Read the model definition and answer for the solid it produces. Units are mm, in the model's axes. Face numbers are marked on the shaded views. A direction names the side the tool comes from. Coordinates: 2 decimals unless noted, no trailing zeros. Write each loop counter-clockwise with the first axis right and the second up, starting at its lowest first coordinate (ties: lowest second). Pieces come first, ordered by that corner, then holes. Notation, with made-up numbers: (15, 12) -> (49, 12) arc R18 ccw to (49, 45) -> close; hole circle Ø3 at (18, 22.25). An arc over 180 degrees is marked (long way). One line per item, written item: value. Start each with the question number.
from build123d import *

# Parameters (mm, degrees)
SKETCH1_R           = 1
SKETCH1_R_2         = 2
BOSS_EXTRUDE1_DEPTH = 44
SKETCH2_W           = 30
SKETCH2_H           = 40
CUT_EXTRUDE1_DEPTH  = 58.965506985
SKETCH3_W           = 5
SKETCH3_H           = 3
BOSS_EXTRUDE2_DEPTH = 20
SKETCH4_R           = 1
CUT_EXTRUDE2_DEPTH  = 62.579217273


with BuildPart() as part:
    # Sketch1 → Boss-Extrude1 (new body)
    with BuildSketch(Plane(origin=(0, 0, 0), x_dir=(1, 0, 0), z_dir=(0, 1, 0))):
        with BuildLine():
            Line((-16, 0), (-16, 20))
            Line((-16, 20), (16, 20))
            Line((16, 20), (16, 0))
            ThreePointArc((16, 0), (0, -16), (-16, 0))
        make_face()
        with Locations(Location((0, 8, 0), (0, 0, 270))):
            Circle(SKETCH1_R, mode=Mode.SUBTRACT)
        with Locations(Location((8, 0, 0), (0, 0, 270))):
            Circle(SKETCH1_R, mode=Mode.SUBTRACT)
        with Locations(Location((0, -8, 0), (0, 0, 270))):
            Circle(SKETCH1_R, mode=Mode.SUBTRACT)
        with Locations(Location((-8, 0, 0), (0, 0, 270))):
            Circle(SKETCH1_R, mode=Mode.SUBTRACT)
        with Locations(Location((0, 0, 0), (0, 0, 270))):
            Circle(SKETCH1_R_2, mode=Mode.SUBTRACT)
    extrude(amount=BOSS_EXTRUDE1_DEPTH)

    # Sketch2 → Cut-Extrude1 (cut, through all)
    with BuildSketch(Plane(origin=(16, 0, 0), x_dir=(0, 0, -1), z_dir=(1, 0, 0))):
        with Locations((-1, 22)):
            Rectangle(SKETCH2_W, SKETCH2_H)
    extrude(amount=-CUT_EXTRUDE1_DEPTH, mode=Mode.SUBTRACT)

    # Sketch3 → Boss-Extrude2 (add)
    with BuildSketch(Plane(origin=(0, 0, -20), x_dir=(-1, 0, 0), z_dir=(0, 0, -1))):
        with Locations((-13.5, 39.5)):
            Rectangle(SKETCH3_W, SKETCH3_H)
        with Locations((13.5, 39.5)):
            Rectangle(SKETCH3_W, SKETCH3_H)
        with Locations((-13.5, 4.5)):
            Rectangle(SKETCH3_W, SKETCH3_H)
        with Locations((13.5, 4.5)):
            Rectangle(SKETCH3_W, SKETCH3_H)
    extrude(amount=BOSS_EXTRUDE2_DEPTH)

    # Sketch4 → Cut-Extrude2 (cut, through all)
    with BuildSketch(Plane.XZ):
        with Locations((-13.5, -27.8)):
            Circle(SKETCH4_R)
        with Locations((-13.5, -35.8)):
            Circle(SKETCH4_R)
        with Locations(Location((13.5, -27.8, 0), (0, 0, 270))):
            Circle(SKETCH4_R)
        with Locations(Location((13.5, -35.8, 0), (0, 0, 270))):
            Circle(SKETCH4_R)
    extrude(amount=-CUT_EXTRUDE2_DEPTH, mode=Mode.SUBTRACT)


solid = part.part
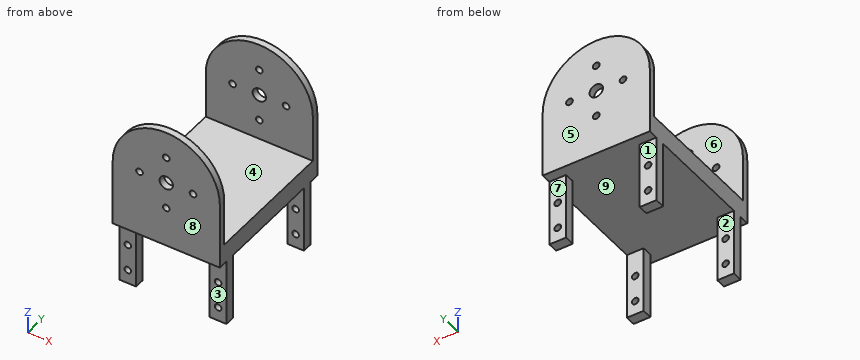
1. A tool of negligible diameter and unlimited length cuts with its end or side. For the marked faces 1, 2, 3, 4 and 5, from which of +Z, -Z, +X, -X, +Y, -Y can it reach the whole face along a straight path? Write none if from no direction.
2. Find the intervals of material crossed by probe 1 along Y at (x, z) = (-9.5, -1); probe 2 along X at (y, z) = (39, -27); probe 3 along Y at (x, z) = (12, -25.5), in increasing order. Write a range as from..to.
3. Given pin 1 (5.5 mm diameter, centred on x = -14, z = -27.5, fed in from -Y); pin 2 (2.5 mm diameter, centred on x = -14.5, z = -27.5, fed in from +Y); pin 3 (6 mm diameter, centred on x = -6.5, y = 36, fed in from -Z), each flat-ended and moving along its own axis, determine where each tip first touches the part or whether it passes through.
4. For a pull along Y with two mould halves and no side action, classify the marked faces 6, 7, 8 and 9 as +Y half, -Y half, draft (parallel to the pull), parting line (faces both ways), or undercut.
5. A cutting plane is placed at C-C on z = -5. Give the vertices of the cut face in (x, y), then the cut area to 3 significant figures.
6. A cutting plane is placed at A-A on z = -27.8. Count the separate pieces of the cut face and the enclosed holes in it, then the cut area to 3 significant figures.
7. A cutting plane is placed at D-D on x = -8. Give the vertices of the cut face in (y, z), then the cut area to 3 significant figures.
8. A cutting plane is placed at B-B on y = 40. Give the vertices of the cut face in (x, z).
Derived:
1. face 1: -Z, +X, -X, +Y
1. face 2: -Z, +X, -X
1. face 3: -Z, +X, -X, -Y
1. face 4: +Z, +X, -X
1. face 5: +Z, -Z, +X, -X, +Y
2. probe 1: y = 0..2, 42..44
2. probe 2: x = -16..-14.1, -12.9..-11, 11..12.9, 14.1..16
2. probe 3: y = 3..6, 38..41
3. pin 1: stops at y = 3
3. pin 2: stops at y = 41
3. pin 3: stops at z = -20
4. face 6: undercut
4. face 7: +Y half
4. face 8: -Y half
4. face 9: undercut
5. outline: (-16, 0) -> (16, 0) -> (16, 2) -> (-16, 2) -> close; (-16, 42) -> (16, 42) -> (16, 44) -> (-16, 44) -> close
5. area: 128 mm2
6. separate pieces: 8
6. enclosed holes: 0
6. area: 36.0 mm2
7. outline: (0, -20) -> (44, -20) -> (44, -1) -> (42, -1) -> (42, -14) -> (2, -14) -> (2, -1) -> (0, -1) -> close; (0, 1) -> (2, 1) -> (2, 13.86) -> (0, 13.86) -> close; (42, 1) -> (44, 1) -> (44, 13.86) -> (42, 13.86) -> close
7. area: 367 mm2
8. outline: (-16, -40) -> (-11, -40) -> (-11, -20) -> (11, -20) -> (11, -40) -> (16, -40) -> (16, -14) -> (-16, -14) -> close; hole circle Ø2 at (-13.5, -35.8); hole circle Ø2 at (-13.5, -27.8); hole circle Ø2 at (13.5, -35.8); hole circle Ø2 at (13.5, -27.8)
